Build history of the part. All positions in model axes, mm. A direction names the side the tool comes from. Give positions to 0.01 mm unless a question says otherwise; leave off trailing zeros. Order: outer loops, then holes, each group sorted by start corner. A loop starts at its lowest first (then second) coordinate and runs counter-clockwise, first axis right, second up. Notation, with made-up numbers: (6, 66.25) - (29, 66.25) arc R19 cw to (29, 76.25) - close; hole circle Ø2 at (5.25, 20.5). An arc over 180 degrees is marked (long way). Use a Markdown table: item, result.
from build123d import *

# Parameters (mm, degrees)
SKETCH1_W           = 3.175
SKETCH1_H           = 63.5
BOSS_EXTRUDE1_DEPTH = 88.9
BOSS_EXTRUDE2_DEPTH = 3.175


with BuildPart() as part:
    # Sketch1 → Boss-Extrude1 (new body)
    with BuildSketch(Plane.XY):
        Rectangle(SKETCH1_W, SKETCH1_H)
    extrude(amount=BOSS_EXTRUDE1_DEPTH)

    # Sketch2 → Boss-Extrude2 (add, symmetric)
    with BuildSketch(Plane(origin=(0, 0, 0), x_dir=(1, 0, 0), z_dir=(0, 1, 0))):
        Polygon((1.5875, 0), (1.5875, 2.2), (4.5847, 2.2), (4.5847, 4.2), (-1.5875, 4.2), (-1.5875, 0), align=None)
    extrude(amount=BOSS_EXTRUDE2_DEPTH, both=True)


solid = part.part
1) Slice it at A-A (x = 0.25). Write the cut outline in (y, z) (3 decimals).
Computed:
| item | result |
|---|---|
| outline | (-31.75, 0) - (-3.175, 0) - (-3.175, -4.2) - (3.175, -4.2) - (3.175, 0) - (31.75, 0) - (31.75, 88.9) - (-31.75, 88.9) - close |
2) Tool access for faces 1 (the flat face through (3, 0, -2.2)), 2 (the flat face through (0, -17, 0)), 3 (the flat face through (0, 18, 0)): list every direction of +Z, -Z, +X, -X, +Y, -Y with a clear straight run to the whole face (end or side of a thin tool).
Computed:
| item | result |
|---|---|
| face 1 | +Z, +X, +Y, -Y |
| face 2 | -Z, +X, -X, -Y |
| face 3 | -Z, +X, -X, +Y |
3) Pin check, flat tips, straight feed: P1, Ø3.5, axis at x = 0.5, y = 13.5, coming from the -Z side; P2, Ø2, axis at x = 2, z = -1.5, coming from the -Y side (3 decimals); P3, Ø3, axis at y = 11, z = 62.5, coming from the +X side. Stop position of each tip, or through.
Computed:
| item | result |
|---|---|
| P1 | stops at z = 0 |
| P2 | stops at y = -3.175 |
| P3 | stops at x = 1.59 |
4) Slice it at B-B (y = 15). Write the cut outline in (x, z), and give its area (3 significant figures).
Computed:
| item | result |
|---|---|
| outline | (-1.59, 0) - (1.59, 0) - (1.59, 88.9) - (-1.59, 88.9) - close |
| area | 282 mm² |
5) Wall check: line 1 (X direction, y = 11.5, z = 64.5); line 2 (Z direction, x = 2, y = 2.5); line 3 (Z direction, x = 1.5, y = 20). Give the ranges that are in metal, low to high. Write a range as from..to.
Computed:
| item | result |
|---|---|
| line 1 | x = -1.59..1.59 |
| line 2 | z = -4.2..-2.2 |
| line 3 | z = 0..88.9 |
6) Slice it at C-C (z = 71.5). Write the cut outline in (x, y).
Computed:
| item | result |
|---|---|
| outline | (-1.59, -31.75) - (1.59, -31.75) - (1.59, 31.75) - (-1.59, 31.75) - close |
